from build123d import *

# Parameters (mm, degrees)
BOSS_EXTRUDE1_DEPTH = 25
SKETCH2_W           = 19.5
SKETCH2_H           = 13
CUT_EXTRUDE1_DEPTH  = 298.867420172
SKETCH3_R           = 2.5
SKETCH3_W           = 14.5
SKETCH3_H           = 12
SKETCH3_H_2         = 27
CUT_EXTRUDE2_DEPTH  = 5
FILLET2_R           = 10
FILLET3_R           = 5
FILLET4_R           = 1


with BuildPart() as part:
    # Sketch1 → Boss-Extrude1 (new, symmetric)
    with BuildSketch(Plane.XY):
        Polygon((-215, 0), (-150, 0), (-150, 180), (150, 180), (150, 0), (215, 0), (215, 15), (165, 15), (165, 195), (165, 200), (150, 200), (-150, 200), (-165, 200), (-165, 195), (-165, 15), (-215, 15), align=None)
    extrude(amount=BOSS_EXTRUDE1_DEPTH, both=True)

    # Sketch2 → Cut-Extrude1 (cut, through all)
    with BuildSketch(Plane.XY.offset(25)):
        with Locations((0, 190)):
            Rectangle(SKETCH2_W, SKETCH2_H)
    extrude(amount=-CUT_EXTRUDE1_DEPTH, mode=Mode.SUBTRACT)

    # Sketch3 → Cut-Extrude2 (cut)
    with BuildSketch(Plane.XZ.offset(-180)):
        with Locations(Location((0, 10, 0), (0, 0, 270))):
            Circle(SKETCH3_R)
        with Locations((0, 19)):
            Rectangle(SKETCH3_W, SKETCH3_H)
        with Locations((0, -6.5)):
            Rectangle(SKETCH3_W, SKETCH3_H_2)
    extrude(amount=-CUT_EXTRUDE2_DEPTH, mode=Mode.SUBTRACT)

    # Fillet2
    fillet2_edges = [part.edges().sort_by_distance(p)[0] for p in [
        (150, 180, 0),
        (-150, 180, 0),
    ]]
    fillet(fillet2_edges, radius=FILLET2_R)

    # Fillet3
    fillet3_edges = [part.edges().sort_by_distance(p)[0] for p in [
        (-215, 15, 0),
        (-165, 15, 0),
        (165, 15, 0),
        (215, 15, 0),
        (150, 0, 0),
        (-150, 0, 0),
    ]]
    fillet(fillet3_edges, radius=FILLET3_R)

    # Fillet4
    fillet4_edges = [part.edges().sort_by_distance(p)[0] for p in [
        (150, 87.5, -25),
        (150, 87.5, 25),
        (-73.625, 180, 25),
        (0, 180, -25),
        (147.071067812, 177.071067812, -25),
        (147.071067812, 177.071067812, 25),
        (-147.071067812, 177.071067812, -25),
        (-147.071067812, 177.071067812, 25),
        (185, 0, -25),
        (185, 0, 25),
        (-215, 5, -25),
        (-190, 15, -25),
        (165, 110, -25),
        (190, 15, -25),
        (-150, 87.5, -25),
        (-213.535533906, 13.535533906, -25),
        (213.535533906, 13.535533906, -25),
        (-151.464466094, 1.464466094, -25),
        (151.464466094, 1.464466094, -25),
        (190, 15, 25),
        (165, 110, 25),
        (-190, 15, 25),
        (-215, 5, 25),
        (-150, 87.5, 25),
        (-213.535533906, 13.535533906, 25),
        (213.535533906, 13.535533906, 25),
        (-151.464466094, 1.464466094, 25),
        (151.464466094, 1.464466094, 25),
        (166.464466094, 16.464466094, -25),
        (166.464466094, 16.464466094, 25),
        (-166.464466094, 16.464466094, -25),
        (-166.464466094, 16.464466094, 25),
        (-165, 110, -25),
        (0, 200, -25),
        (215, 5, -25),
        (-185, 0, -25),
        (215, 5, 25),
        (0, 200, 25),
        (9.75, 190, -25),
        (0, 183.5, -25),
        (-9.75, 190, -25),
        (0, 196.5, -25),
        (9.75, 190, 25),
        (0, 196.5, 25),
        (-9.75, 190, 25),
        (-8.5, 183.5, 25),
        (-165, 110, 25),
        (8.5, 183.5, 25),
        (73.625, 180, 25),
        (-7.25, 181.75, 25),
        (7.25, 181.75, 25),
        (-185, 0, 25),
    ]]
    fillet(fillet4_edges, radius=FILLET4_R)


solid = part.part
Verification items for the finished model (mm, model axes). A direction names the side the tool comes from. Round coordinates to 2 decimals unless told otherwise and drop trailing zeros. Loops run counter-clockwise (first coordinate to the right, second up) from the corner with the lowest first, then second, coordinate; pieces in that order, holes last. Notation, with made-up numbers: (21, 18) - (45, 18) arc R10 ccw to (45, 24) - close; hole circle Ø7 at (-28.5, 25.5). An arc over 180 degrees is marked (long way). Answer in a Markdown table with one row per item. Add a question column.
Q1. Material ranges on line 1 (X direction, y = 41.5, z = 15); line 2 (X direction, y = 182.8, z = 10); line 3 (Y direction, x = -69.5, z = -11.5), recorded low to high.
Q2. Section check A-A on y = 54.5. Enter the section's corners in (x, z), plus the area to 3 significant figures.
Q3. Section check B-B on x = 18.5. Enter the section's corners in (y, z).
Q4. Tool access check on faces 1 (the face through (-165, 111, 0)), 2 (the face through (-185, 0, 0)), 3 (the face through (-9, 183.5, -5)), 4 (the face through (-147.15, 176.99, 0.34)). Record the directions out of +Z, -Z, +X, -X, +Y, -Y that give a thin tool (end or side, any length) a straight path to the whole face; none if there is none.
Q5. Release check for a two-part mould opening along Y. For faces 5 (the face through (150, 89, 0)), 6 (the face through (146.99, 177.15, 0.34)), 7 (the face through (-190, 15, 0)), 8 (the face through (-9.75, 190, 0)) record: pulls with the +Y half, pulls with the -Y half, needs draft (parallel to the pull), parting line crosses it, or undercut.
Q6. Section check C-C on z = -5.5. Enter the section's corners in (x, y), plus the area to 3 significant figures.
Q7. Gauge pin test, flat ends, axial feed: pin 1 (6 mm diameter, centred on y = 134.5, z = 17.5, fed in from +X); pin 2 (3 mm diameter, centred on x = 1.5, y = 181.5, fed in from +Z); pin 3 (6 mm diameter, centred on x = 0, z = 10, fed in from -Y). Record the tip position at first contact, or that the pin passes through.
Found:
| question | item | result |
|---|---|---|
| 1 | line 1 | x = -165 to -150, 150 to 165 |
| 1 | line 2 | x = -165 to -2.5, 2.5 to 165 |
| 1 | line 3 | y = 180 to 200 |
| 2 | outline | (-165, -24) arc R1 ccw to (-164, -25) - (-151, -25) arc R1 ccw to (-150, -24) - (-150, 24) arc R1 ccw to (-151, 25) - (-164, 25) arc R1 ccw to (-165, 24) - close; (150, -24) arc R1 ccw to (151, -25) - (164, -25) arc R1 ccw to (165, -24) - (165, 24) arc R1 ccw to (164, 25) - (151, 25) arc R1 ccw to (150, 24) - close |
| 2 | area | 1,500 mm² |
| 3 | outline | (180, -24) arc R1 ccw to (181, -25) - (199, -25) arc R1 ccw to (200, -24) - (200, 24) arc R1 ccw to (199, 25) - (181, 25) arc R1 ccw to (180, 24) - close |
| 4 | face 1 | +Z, -Z, -X, +Y |
| 4 | face 2 | +Z, -Z, +X, -X, -Y |
| 4 | face 3 | +Z, -Z |
| 4 | face 4 | +Z, -Z, -Y |
| 5 | face 5 | needs draft |
| 5 | face 6 | pulls with the -Y half |
| 5 | face 7 | pulls with the +Y half |
| 5 | face 8 | undercut |
| 6 | outline | (-215, 0) - (-155, 0) arc R5 ccw to (-150, 5) - (-150, 170) arc R10 cw to (-140, 180) - (-7.25, 180) - (-7.25, 183.5) - (-9.75, 183.5) - (-9.75, 196.5) - (9.75, 196.5) - (9.75, 183.5) - (7.25, 183.5) - (7.25, 180) - (140, 180) arc R10 cw to (150, 170) - (150, 5) arc R5 ccw to (155, 0) - (215, 0) - (215, 10) arc R5 ccw to (210, 15) - (170, 15) arc R5 cw to (165, 20) - (165, 200) - (-165, 200) - (-165, 20) arc R5 cw to (-170, 15) - (-210, 15) arc R5 ccw to (-215, 10) - close |
| 6 | area | 13,200 mm² |
| 7 | pin 1 | stops at x = 165 |
| 7 | pin 2 | stops at z = 13 |
| 7 | pin 3 | stops at y = 180 |
